For this review, take the finished solid that the model builds, in its own axes (mm). Face numbers are marked on the shaded views. A direction names the side the tool comes from. Round coordinates to 2 decimals unless told otherwise and drop trailing zeros. Loops run counter-clockwise (first coordinate to the right, second up) from the corner with the lowest first, then second, coordinate; pieces in that order, holes last.
1. Consider section B-B on x = 0. State the section outline as (y, z) points.
2. To check wall thickness, follow line 1 along Z through (x, y) = (0, -7.65); line 2 along Z through (x, y) = (32, -4); line 3 along Y through (x, z) = (-0.5, 1). State the ranges of each line that lie inside material, in increasing order.
3. Tool access review of the marked faces 4, 5 and 6: name each direction out of +Z, -Z, +X, -X, +Y, -Y from which nothing blocks a thin tool from reaching the whole face with its end or side.
4. Consider section A-A on z = 0. State the section outline as (x, y) points, then the cut area to 3 significant figures.
5. Consider section C-C on x = 9. State the section outline as (y, z) points, then the cut area to 3 significant figures.
6. Consider section D-D on z = -16. State the section outline as (x, y) points.
7. Clearance check with flat-ended pins moving along their axes: pin 1 Ø1.5 at (y, z) = (-4.5, -8.5) entering from +X; pin 2 Ø5 at (y, z) = (-6.5, -21.5) entering from -X; pin 3 Ø6 at (x, y) = (27, -7) entering from -Z. State where each tip first meets the part, or that it passes through.
8. Draft analysis for pull direction X (two halves, no side actions). For the marked faces 1, 2 and 3, state which applies: released by +X, released by -X, zero draft, split by the parting line, or undercut.
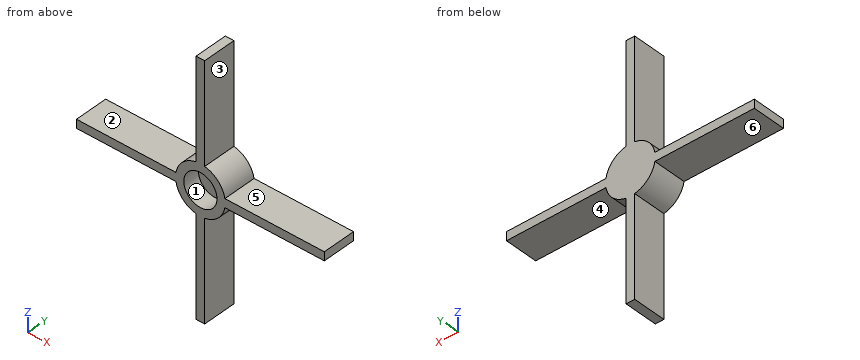
from build123d import *

# Parameters (mm, degrees)
F1_DEPTH = 10
F2_R     = 5
F3_DEPTH = 5


with BuildPart() as f1:
    # F0 (on Front) → F1 (new body)
    with BuildSketch(Plane.XZ):
        with BuildLine():
            ThreePointArc((7.386474, -1.3), (7.471565, -0.652474), (7.5, 0))
            ThreePointArc((7.5, 0), (7.471565, 0.652474), (7.386474, 1.3))
            ThreePointArc((7.386474, 1.3), (5.303301, 5.303301), (1.3, 7.386474))
            ThreePointArc((1.3, 7.386474), (0, 7.5), (-1.3, 7.386474))
            ThreePointArc((-1.3, 7.386474), (-5.303301, 5.303301), (-7.386474, 1.3))
            ThreePointArc((-7.386474, 1.3), (-7.5, 0), (-7.386474, -1.3))
            ThreePointArc((-7.386474, -1.3), (-5.303301, -5.303301), (-1.3, -7.386474))
            ThreePointArc((-1.3, -7.386474), (0, -7.5), (1.3, -7.386474))
            ThreePointArc((1.3, -7.386474), (5.303301, -5.303301), (7.386474, -1.3))
        make_face()
        with BuildLine():
            ThreePointArc((7.386474, 1.3), (7.471565, 0.652474), (7.5, 0))
            ThreePointArc((7.5, 0), (7.471565, -0.652474), (7.386474, -1.3))
            Line((7.386474, -1.3), (37.386474, -1.3))
            Line((37.386474, -1.3), (37.386474, 0))
            Line((37.386474, 0), (37.386474, 1.3))
            Line((37.386474, 1.3), (7.386474, 1.3))
        make_face()
        with BuildLine():
            ThreePointArc((-1.3, 7.386474), (0, 7.5), (1.3, 7.386474))
            Line((1.3, 7.386474), (1.3, 37.5))
            Line((1.3, 37.5), (0, 37.5))
            Line((0, 37.5), (-1.3, 37.5))
            Line((-1.3, 37.5), (-1.3, 7.386474))
        make_face()
        with BuildLine():
            Line((1.3, -37.5), (1.3, -7.386474))
            ThreePointArc((1.3, -7.386474), (0, -7.5), (-1.3, -7.386474))
            Line((-1.3, -7.386474), (-1.3, -37.5))
            Line((-1.3, -37.5), (0, -37.5))
            Line((0, -37.5), (1.3, -37.5))
        make_face()
        with BuildLine():
            ThreePointArc((-7.386474, -1.3), (-7.5, 0), (-7.386474, 1.3))
            Line((-7.386474, 1.3), (-37.386474, 1.3))
            Line((-37.386474, 1.3), (-37.386474, 0))
            Line((-37.386474, 0), (-37.386474, -1.3))
            Line((-37.386474, -1.3), (-7.386474, -1.3))
        make_face()
    extrude(amount=F1_DEPTH)

    # F2 (on face) → F3 (cut)
    with BuildSketch(Plane.XZ.offset(10)):
        Circle(F2_R)
    extrude(amount=-F3_DEPTH, mode=Mode.SUBTRACT)


solid = f1.part
Resolved:
1. outline: (-10, -37.5) - (0, -37.5) - (0, 37.5) - (-10, 37.5) - (-10, 5) - (-5, 5) - (-5, -5) - (-10, -5) - close
2. line 1: z = -37.5 to -5, 5 to 37.5
2. line 2: z = -1.3 to 1.3
2. line 3: y = -5 to 0
3. face 4: -Z, +X, +Y, -Y
3. face 5: +Z, +X, +Y, -Y
3. face 6: -Z, -X, +Y, -Y
4. outline: (-37.39, -10) - (-5, -10) - (-5, -5) - (5, -5) - (5, -10) - (37.39, -10) - (37.39, 0) - (-37.39, 0) - close
4. area: 698 mm2
5. outline: (-10, -1.3) - (0, -1.3) - (0, 1.3) - (-10, 1.3) - close
5. area: 26.0 mm2
6. outline: (-1.3, -10) - (1.3, -10) - (1.3, 0) - (-1.3, 0) - close
7. pin 1: stops at x = 1.3
7. pin 2: stops at x = -1.3
7. pin 3: stops at z = -1.3
8. face 1: undercut
8. face 2: zero draft
8. face 3: released by +X
